Verification items for the finished model (mm, model axes). Coordinates: 2 decimals unless noted, no trailing zeros. Write each loop counter-clockwise with the first axis right and the second up, starting at its lowest first coordinate (ties: lowest second). Pieces come first, ordered by that corner, then holes. Notation, with made-up numbers: M 40,86 L 88,86 A6 cw 88,97 Z; hole C 65,74 d3. An arc over 180 degrees is marked long. One line per item, written item: value.
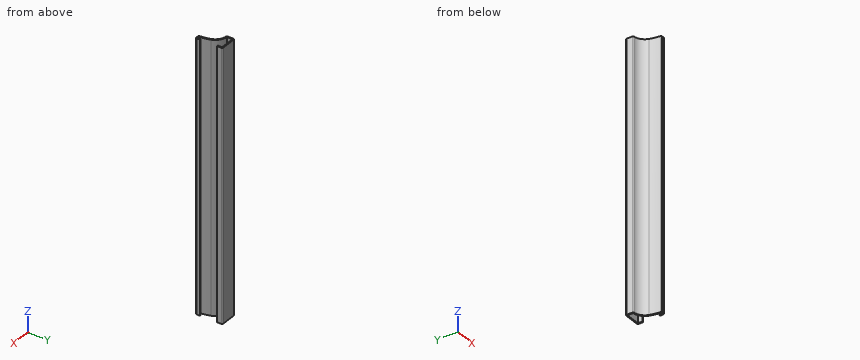
```python
from build123d import *

# Parameters (mm, degrees)
EXTRUDE_THIN1_DEPTH = 301.625
FILLET1_R           = 1.27


with BuildPart() as part:
    # Sketch1 → Extrude-Thin1 (new body)
    with BuildSketch(Plane.XY):
        with BuildLine():
            Line((0, 0), (0, 6.35))
            Line((0, 6.35), (-19.05, 6.35))
            Line((-19.05, 6.35), (-19.05, -2.38125))
            ThreePointArc((-19.05, -2.38125), (-11.575450433, -4.813771791), (-6.964208693, -11.179500588))
            ThreePointArc((-6.964208693, -11.179500588), (-5.421346287, -17.418966095), (-4.7625, -23.8125))
            Line((-4.7625, -23.8125), (0, -23.8125))
            Line((0, -23.8125), (0, -19.05))
            Line((0, -19.05), (-1.27, -19.05))
            Line((-1.27, -19.05), (-1.27, -22.5425))
            Line((-1.27, -22.5425), (-3.549505015, -22.5425))
            ThreePointArc((-3.549505015, -22.5425), (-4.279699966, -16.595923923), (-5.755629562, -10.789325647))
            ThreePointArc((-5.755629562, -10.789325647), (-10.322605132, -4.172836787), (-17.78, -1.169097039))
            Line((-17.78, -1.169097039), (-17.78, 5.08))
            Line((-17.78, 5.08), (-1.27, 5.08))
            Line((-1.27, 5.08), (-1.27, 0))
            Line((-1.27, 0), (0, 0))
        make_face()
    extrude(amount=-EXTRUDE_THIN1_DEPTH)

    # Fillet1
    fillet1_edges = [part.edges().sort_by_distance(p)[0] for p in [
        (0, -23.8125, -150.8125),
        (-4.7625, -23.8125, -150.8125),
        (-19.05, -2.38125, -150.8125),
        (-19.05, 6.35, -150.8125),
        (0, 6.35, -150.8125),
    ]]
    fillet(fillet1_edges, radius=FILLET1_R)


solid = part.part
```
Item 1: Scan lines: line 1 (Y direction, x = -2, z = -195.5); line 2 (X direction, y = 2, z = -216); line 3 (Y direction, x = -1, z = -15.5). Record each from-to range of solid material in increasing order.
The answers:
line 1: y = -23.81 to -22.54, 5.08 to 6.35
line 2: x = -19.05 to -17.78, -1.27 to 0
line 3: y = -23.78 to -19.05, 0 to 6.32
Item 2: Cross-section at C-C, the plane y = -6. Enter the section's corners in (x, z) (3 decimals).
The answers:
outline: M -10.172,-301.625 L -8.434,-301.625 L -8.434,0 L -10.172,0 Z
Item 3: Cross-section at A-A, the plane x = -14. Enter the section's corners in (y, z) (3 decimals).
The answers:
outline: M -3.428,-301.625 L -2.056,-301.625 L -2.056,0 L -3.428,0 Z; M 5.08,-301.625 L 6.35,-301.625 L 6.35,0 L 5.08,0 Z
Item 4: Go/stop test with flat-tipped pins: P1, Ø1, axis at y = -17.5, z = -249, coming from the -X side; P2, Ø3, axis at y = -11.5, z = -99.5, coming from the +X side; P3, Ø6, axis at x = -15.5, z = -198.5, coming from the -Y side; P4, Ø1.4, axis at x = -0.5, z = -100, coming from the +Y side. Record where each tip stops, or that it passes through.
The answers:
P1: stops at x = -5.5
P2: stops at x = -5.1
P3: stops at y = -4.2
P4: stops at y = 6.35
